from build123d import *

# Parameters (mm, degrees)
IZIM1_W                     = 40
IZIM1_H                     = 0.6
Y_KSEKLIK_EKSTR_ZYON1_DEPTH = 12
IZIM2_R                     = 2.7
KES_EKSTR_ZYON1_DEPTH       = 42.992380261
RADYUS1_R                   = 1.5
RADYUS2_R                   = 0.5


with BuildPart() as part:
    # Çizim1 → Yükseklik-Ekstrüzyon1 (new body)
    with BuildSketch(Plane(origin=(0, 0, 0), x_dir=(0, 0, -1), z_dir=(1, 0, 0))):
        Polygon((28, 0), (12, 0), (12, -2.1), (14, -2.1), (14.981495458, -3.8), (25.018504542, -3.8), (26, -2.1), (28, -2.1), align=None)
        Polygon((12, 2.7), (12, 0.6), (28, 0.6), (28, 2.7), (26, 2.7), (25.018504542, 4.4), (14.981495458, 4.4), (14, 2.7), align=None)
        with Locations((20, 0.3)):
            Rectangle(IZIM1_W, IZIM1_H)
    extrude(amount=Y_KSEKLIK_EKSTR_ZYON1_DEPTH)

    # Çizim2 → Kes-Ekstrüzyon1 (cut, through all)
    with BuildSketch(Plane(origin=(0, 0.6, 0), x_dir=(1, 0, 0), z_dir=(0, 1, 0))):
        with Locations(Location((6, 5, 0), (0, 0, 270))):
            Circle(IZIM2_R)
        with Locations(Location((6, 35, 0), (0, 0, 270))):
            Circle(IZIM2_R)
    extrude(amount=-KES_EKSTR_ZYON1_DEPTH, mode=Mode.SUBTRACT)

    # Radyus1
    radyus1_edges = [part.edges().sort_by_distance(p)[0] for p in [
        (12, 0.3, -40),
        (0, 0.3, 0),
        (0, 0.3, -40),
        (12, 0.3, 0),
    ]]
    fillet(radyus1_edges, radius=RADYUS1_R)

    # Radyus2
    radyus2_edges = [part.edges().sort_by_distance(p)[0] for p in [
        (6, -2.1, -28),
        (6, -2.1, -26),
        (6, -3.8, -25.018504542),
        (6, -3.8, -14.981495458),
        (6, -2.1, -14),
        (6, -2.1, -12),
        (6, 0, -12),
        (6, 0.6, -12),
        (6, 2.7, -12),
        (6, 2.7, -14),
        (6, 4.4, -14.981495458),
        (6, 4.4, -25.018504542),
        (6, 2.7, -26),
        (6, 2.7, -28),
        (6, 0.6, -28),
        (6, 0, -28),
    ]]
    fillet(radyus2_edges, radius=RADYUS2_R)


solid = part.part
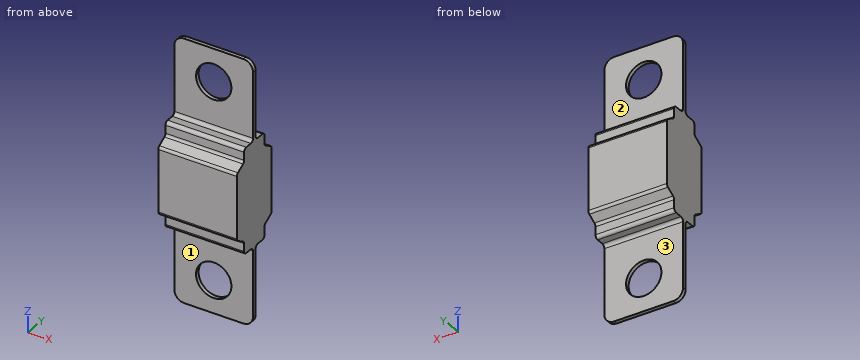
Check sheet for the modelled part. Datum: model origin and axes. Units: mm. Face numbers are marked on the shaded views. A direction names the side the tool comes from. Coordinates: 2 decimals unless noted, no trailing zeros. Write each loop counter-clockwise with the first axis right and the second up, starting at its lowest first coordinate (ties: lowest second). Pieces come first, ordered by that corner, then holes.
Item 1: Cross-section at D-D on y = -2.75. Record the boundary of the cut face in (x, z), then the cut area to 3 significant figures.
Numbers:
outline: (0, -25.62) - (12, -25.62) - (12, -14.38) - (0, -14.38) - close
area: 135 mm2
Item 2: Depth check by flat-ended pin: pin 1 Ø1.3 at (x, z) = (5.5, -13) entering from +Y; pin 2 Ø1.2 at (x, y) = (3.5, -1.5) entering from +Z; pin 3 Ø6 at (x, z) = (7, -6) entering from -Y; pin 4 Ø4 at (x, y) = (10.5, -1) entering from -Z. Enter the tip coordinate at first touch or a pass-through.
Numbers:
pin 1: stops at y = 2.7
pin 2: stops at z = -12
pin 3: stops at y = 0
pin 4: stops at z = -40
Item 3: Scan lines: probe 1 along X at (y, z) = (0.2, -5); probe 2 along Y at (x, z) = (9, -1.5); probe 3 along Z at (x, y) = (4.5, 0.25) (3 decimals). Record each from-to range of solid material in increasing order.
Numbers:
probe 1: x = 0 to 3.3, 8.7 to 12
probe 2: y = 0 to 0.6
probe 3: z = -40 to -37.245, -32.755 to -7.245, -2.755 to 0
Item 4: Cross-section at B-B on x = 6. Count the separate pieces of the cut face and the enclosed holes in it, then the cut area to 3 significant figures.
Numbers:
separate pieces: 3
enclosed holes: 0
area: 122 mm2
Item 5: Access from +Z, -Z, +X, -X, +Y, -Y to the whole of each face (thin tool, end or side, straight path). Record for the marked faces 1, 2 and 3.
Numbers:
face 1: -Z, +X, -X, -Y
face 2: +Z, +X, -X, +Y
face 3: -Z, +X, -X, +Y
Item 6: Cross-section at A-A on z = -5. Record the boundary of the cut face in (x, y).
Numbers:
outline: (0, 0) - (3.3, 0) - (3.3, 0.6) - (0, 0.6) - close; (8.7, 0) - (12, 0) - (12, 0.6) - (8.7, 0.6) - close
Item 7: Cross-section at C-C on z = -31. Record the boundary of the cut face in (x, y).
Numbers:
outline: (0, 0) - (12, 0) - (12, 0.6) - (0, 0.6) - close
